Model file for the job. Use its own axes, mm. A direction names the side the tool comes from. Give positions to 0.01 mm unless a question says otherwise; leave off trailing zeros. Loops run counter-clockwise (first coordinate to the right, second up) from the corner with the lowest first, then second, coordinate; pieces in that order, holes last. Notation, with made-up numbers: M 47,10.25 L 71,10.25 A20 ccw 71,18.25 Z; hole C 75.5,-34.75 d11. An arc over 180 degrees is marked long. Answer in a Markdown table with one row per item.
Autodesk Inventor part; units mm, degrees
ref_plane "YZ Plane" through (0, 0, 0) normal (1, 0, 0) x (0, 1, 0)
ref_plane "XZ Plane" through (0, 0, 0) normal (0, 1, 0) x (-1, 0, 0)
ref_plane "XY Plane" through (0, 0, 0) normal (0, 0, 1) x (1, 0, 0)
sketch "Sketch1" plane through (0, 0, 0) normal (0, 1, 0) x (-1, 0, 0)
  circle A0 centre (0, 0) radius 4.55
  dimension "d0" = 9.1
extrude "Extrusion1" add sketch "Sketch1" along normal blind 1.52
sketch "Sketch2" plane through (0, 1.52, 0) normal (0, 1, 0) x (1, 0, 0)
  line L0 (2.47, -2.465) -> (-2.47, -2.465)
  line L1 (-2.47, -2.465) -> (-2.47, 2.465)
  line L2 (-2.47, 2.465) -> (2.47, 2.465)
  line L3 (2.47, 2.465) -> (2.47, -2.465)
  line L4 (2.47, -2.465) -> (-2.47, 2.465) construction
  line L5 (-2.47, -2.465) -> (2.47, 2.465) construction
  point P0 (0, 0)
  dimension "d3" = 4.94
  dimension "d4" = 4.93
extrude "Extrusion2" add sketch "Sketch2" along normal blind 1.5
sketch "Sketch3" plane through (0, 1.52, 0) normal (0, 1, 0) x (1, 0, 0)
  line L0 (3.935, 1.2) -> (3.085, 1.2)
  line L1 (3.085, 1.2) -> (3.085, -1.2)
  line L2 (3.085, -1.2) -> (3.935, -1.2)
  line L3 (3.935, -1.2) -> (3.935, 1.2)
  line L4 (2.47, -2.465) -> (2.47, 2.465)
  circle A0 centre (0, 0) radius 4.55
  line L5 (0, 4.55) -> (0, -4.55) construction
  line L6 (-3.935, 1.2) -> (-3.085, 1.2)
  line L7 (-3.085, 1.2) -> (-3.085, -1.2)
  line L8 (-3.085, -1.2) -> (-3.935, -1.2)
  line L9 (-3.935, -1.2) -> (-3.935, 1.2)
  dimension "d7" = 2.4
  dimension "d8" = 0.85
  dimension "d9" = 0.615
  dimension "d10" = 0.615
  dimension "d11" = 1.2
  dimension "d12" = 1.2
extrude "Extrusion3" add sketch "Sketch3" along normal blind 0.6 contours L3 L2 L1 L0 | L6 L7 L8 L9
equation "\"d9\" = d10"
equation "\"d11\" = d12"
properties part number "neopixel mini pcb footprint"
Q1. Probe probe 1 along X at (y, z) = (2.65, -2); probe 2 along Y at (x, z) = (0, 2.75); probe 3 along Z at (x, y) = (1.5, 1.75) (3 decimals). List the from-to ranges inside material, lowest first.
Reported:
| item | result |
|---|---|
| probe 1 | -2.47 to 2.47 |
| probe 2 | 0 to 1.52 |
| probe 3 | -2.465 to 2.465 |
Q2. Saw through at A-A (x = 0). Give the cut face in (y, z) (3 decimals), and give its area (3 significant figures).
Reported:
| item | result |
|---|---|
| outline | M 0,-4.55 L 1.52,-4.55 L 1.52,-2.465 L 3.02,-2.465 L 3.02,2.465 L 1.52,2.465 L 1.52,4.55 L 0,4.55 Z |
| area | 21.2 mm² |
Q3. 3-axis set-ups, long thin cutter, end or side, ignore diameter. For faces 1 (the face through (0, 2, -2.465)), 2 (the face through (-3.5, 2.12, 0)), 3 (the face through (-2.47, 2, 0)): which of +Z, -Z, +X, -X, +Y, -Y reach the whole face in a straight line?
Reported:
| item | result |
|---|---|
| face 1 | -Z, +X, -X, +Y |
| face 2 | +Z, -Z, -X, +Y |
| face 3 | +Z, -Z, +Y |
Q4. Saw through at C-C (y = 2.45). Give the cut face in (x, z) (3 decimals).
Reported:
| item | result |
|---|---|
| outline | M -2.47,-2.465 L 2.47,-2.465 L 2.47,2.465 L -2.47,2.465 Z |
Q5. Saw through at B-B (z = 0). Give the cut face in (x, y) (3 decimals), and give its area (3 significant figures).
Reported:
| item | result |
|---|---|
| outline | M -4.55,0 L 4.55,0 L 4.55,1.52 L 3.935,1.52 L 3.935,2.12 L 3.085,2.12 L 3.085,1.52 L 2.47,1.52 L 2.47,3.02 L -2.47,3.02 L -2.47,1.52 L -3.085,1.52 L -3.085,2.12 L -3.935,2.12 L -3.935,1.52 L -4.55,1.52 Z |
| area | 22.3 mm² |
Q6. Drop flat-ended pins along their axis: pin 1 (1.6 mm diameter, centred on y = 2.5, z = 0.5, fed in from -X) (3 decimals); pin 2 (0.5 mm diameter, centred on y = 1.5, z = -0.5, fed in from -X); pin 3 (0.9 mm diameter, centred on x = 3.5, z = 0, fed in from +Y). Give the stop position or say it passes through.
Reported:
| item | result |
|---|---|
| pin 1 | x = -3.935 |
| pin 2 | x = -4.54 |
| pin 3 | y = 2.12 |
Q7. Saw through at D-D (x = -1.75). Give the cut face in (y, z) (3 decimals).
Reported:
| item | result |
|---|---|
| outline | M 0,-4.2 L 1.52,-4.2 L 1.52,-2.465 L 3.02,-2.465 L 3.02,2.465 L 1.52,2.465 L 1.52,4.2 L 0,4.2 Z |
